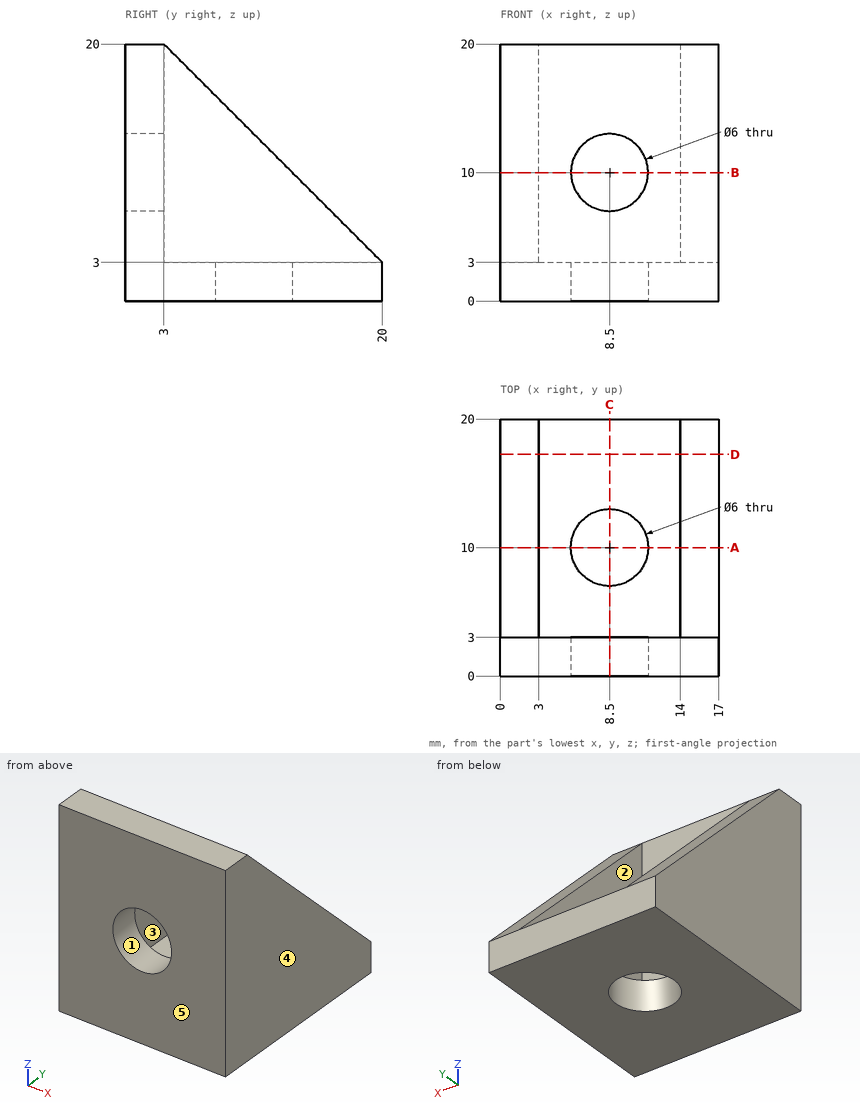
Study the drawing (mm; zero at the part's minimum x, y, z) and answer. A direction names the side the tool comes from. Round coordinates to 2 decimals unless told otherwise and drop trailing zeros. Write each loop counter-clockwise with the first axis right and the second up, starting at its lowest first coordinate (ties: lowest second). Pieces come first, ordered by that corner, then holes. Notation, with made-up numbers: (14, 0) -> (70, 0) arc R20 cw to (70, 23) -> close; hole circle Ø11 at (60, -17). An arc over 180 degrees is marked (long way). Use CSV: the item, a comma, the result in double quotes. Start each with the question number.
(1) Which of the six approach directions +Z, -Z, +X, -X, +Y, -Y give full straight-line access (tool end or side, diameter ignored) to the marked faces 1 and 2?
(2) Consider L1, parallel to X at y = 10, z = 0.9; L2, parallel to Z at x = 8.5, y = 1.4; L3, parallel to X at y = 8.5, z = 4. Determine where each line is inside the solid, lowest interval first. Write a range as from..to.
(3) Section D-D on y = 17.25 is taken. Give the vertices of the cut face in (x, z).
(4) The mould has two halves that part along X. Classify the marked faces 3, 4 and 5: released by +X, released by -X, zero draft, split by the parting line, or undercut.
(5) Section C-C on x = 8.5 is taken. Give the vertices of the cut face in (y, z), then the cut area to 3 significant figures.
(6) Each of these flat-tipped pins is pushed along its axis until it touches: pin 1 (1 mm diameter, centred on x = 5.5, z = 8.5, fed in from +Y); pin 2 (3 mm diameter, centred on x = 6.5, y = 12, fed in from +Z); pin 3 (5.5 mm diameter, centred on x = 8.5, y = 10, fed in from +Z). Where does it stop, or does it pass through?
(7) Section A-A on y = 10 is taken. Give the vertices of the cut face in (x, z), then the cut area to 3 significant figures.
A:
1,face 1,"+Y, -Y"
1,face 2,"+Z, +Y"
2,L1,"x = 0..5.5, 11.5..17"
2,L2,"z = 0..7, 13..20"
2,L3,"x = 0..3, 14..17"
3,outline,"(0, 0) -> (17, 0) -> (17, 5.75) -> (14, 5.75) -> (14, 3) -> (3, 3) -> (3, 5.75) -> (0, 5.75) -> close"
4,face 3,"undercut"
4,face 4,"released by +X"
4,face 5,"zero draft"
5,outline,"(0, 0) -> (7, 0) -> (7, 3) -> (3, 3) -> (3, 7) -> (0, 7) -> close; (0, 13) -> (3, 13) -> (3, 20) -> (0, 20) -> close; (13, 0) -> (20, 0) -> (20, 3) -> (13, 3) -> close"
5,area,"75.0 mm²"
6,pin 1,"stops at y = 3"
6,pin 2,"stops at z = 3"
6,pin 3,"passes through"
7,outline,"(0, 0) -> (5.5, 0) -> (5.5, 3) -> (3, 3) -> (3, 13) -> (0, 13) -> close; (11.5, 0) -> (17, 0) -> (17, 13) -> (14, 13) -> (14, 3) -> (11.5, 3) -> close"
7,area,"93.0 mm²"
